```python
from build123d import *

# Parameters (mm, degrees)
RESSALTO_EXTRUS_O1_DEPTH = 1.4
ESBO_O2_R                = 3.45
RESSALTO_EXTRUS_O2_DEPTH = 2.4
FURO4_D                  = 1.2
PADR_O_LINEAR1_COUNT     = 6
PADR_O_LINEAR1_PITCH     = 2
FURO1_D                  = 4.95
FURO1_DEPTH              = 2
FURO2_D                  = 4.6
FURO2_DEPTH              = 1
FURO3_D                  = 2.1


with BuildPart() as part:
    # Esboço1 → Ressalto-extrusão1 (new body)
    with BuildSketch(Plane(origin=(0, 0, 0), x_dir=(1, 0, 0), z_dir=(0, 1, 0))):
        with BuildLine():
            Line((-14.159121967, 1.99702088), (-2.209072203, 2.65))
            ThreePointArc((-2.209072203, 2.65), (3.45, 0), (-2.209072203, -2.65))
            Line((-2.209072203, -2.65), (-14.159121967, -1.99702088))
            ThreePointArc((-14.159121967, -1.99702088), (-16.05, 0), (-14.159121967, 1.99702088))
        make_face()
    extrude(amount=-RESSALTO_EXTRUS_O1_DEPTH)

    # Esboço2 → Ressalto-extrusão2 (add)
    with BuildSketch(Plane.XZ.offset(1.4)):
        with Locations(Location((0, 0, 0), (0, 0, 90))):
            Circle(ESBO_O2_R)
    extrude(amount=RESSALTO_EXTRUS_O2_DEPTH)

    # Furo4 (through all)
    with Locations(Plane(origin=(0, 0, 0), x_dir=(1, 0, 0), z_dir=(0, 1, 0))):
        with Locations((-14.45, 0)):
            furo4 = Hole(FURO4_D / 2)

    # Padrão linear1: Furo4 ×6
    with Locations(*[(i * PADR_O_LINEAR1_PITCH, 0, 0) for i in range(1, PADR_O_LINEAR1_COUNT)]):
        add(furo4, mode=Mode.SUBTRACT)

    # Furo1
    with Locations(Plane(origin=(0, -3.8, 0), x_dir=(-1, 0, 0), z_dir=(0, -1, 0))):
        with Locations((0, 0)):
            Hole(FURO1_D / 2, depth=FURO1_DEPTH)

    # Furo2
    with Locations(Plane(origin=(0, 0, 0), x_dir=(1, 0, 0), z_dir=(0, 1, 0))):
        with Locations((0, 0)):
            Hole(FURO2_D / 2, depth=FURO2_DEPTH)

    # Furo3 (through all)
    with Locations(Plane(origin=(0, 0, 0), x_dir=(1, 0, 0), z_dir=(0, 1, 0))):
        with Locations((0, 0)):
            Hole(FURO3_D / 2)


solid = part.part
```
Here's how the part is built. I have some questions about the finished solid (model axes, mm). A direction names the side the tool comes from. Coordinates: 2 decimals unless noted, no trailing zeros. Order: outer loops, then holes, each group sorted by start corner. A loop starts at its lowest first (then second) coordinate and runs counter-clockwise, first axis right, second up. Notation, with made-up numbers: (86.25, 30.5) -> (137.25, 30.5) arc R4 cw to (137.25, 35.5) -> close; hole circle Ø8 at (43, 32). An arc over 180 degrees is marked (long way). Return JSON: item names as keys, results as strings.
1) If we section it at B-B on x = -6.45: List the corners of the cut face in (y, z) for me, plus the area to 3 significant figures.
Conclusion:
{"outline": "(-1.4, -2.42) -> (0, -2.42) -> (0, -0.6) -> (-1.4, -0.6) -> close; (-1.4, 0.6) -> (0, 0.6) -> (0, 2.42) -> (-1.4, 2.42) -> close", "area": "5.09 mm²"}
2) If we section it at D-D on z = 1.25: List the corners of the cut face in (x, y) for me, plus the area to 3 significant figures.
Conclusion:
{"outline": "(-15.61, -1.4) -> (-3.22, -1.4) -> (-3.22, -3.8) -> (-2.14, -3.8) -> (-2.14, -1.8) -> (2.14, -1.8) -> (2.14, -3.8) -> (3.22, -3.8) -> (3.22, 0) -> (1.93, 0) -> (1.93, -1) -> (-1.93, -1) -> (-1.93, 0) -> (-15.61, 0) -> close", "area": "29.4 mm²"}
3) If I drill on probe 1 along Z at (x, y) = (0, -0.2); probe 2 along Y at (x, z) = (1.5, 1); probe 3 along X at (y, z) = (-3.6, -1.25), over which ranges is the centre line in solid material (lowest first)?
Conclusion:
{"probe 1": "z = -3.45 to -2.3, 2.3 to 3.45", "probe 2": "y = -1.8 to -1", "probe 3": "x = -3.22 to -2.14, 2.14 to 3.22"}
4) Thinking about a two-plate mould opening in Z: for faces 4 (the cylindrical face through (2.36, -2.79, -0.74)), 5 (the cylindrical face through (-16.05, -0.69, 0.04)), 6 (the flat face through (-9, -1.4, 1)), 7 (the cylindrical face through (-15.004, -0.71, 0.23)), which applies, +Z half, -Z half, draft (parallel to the pull), parting line (faces both ways), or undercut?
Conclusion:
{"face 4": "undercut", "face 5": "parting line", "face 6": "draft", "face 7": "undercut"}
5) On a 3-axis mill with a long thin cutter (end or side, diameter ignored), from which of +Z, -Z, +X, -X, +Y, -Y can I reach the whole of each face in a straight line? I mean faces 1 (the cylindrical face through (-9.004, -0.71, 0.23)), 2 (the flat face through (1, -1.8, 1)), 3 (the cylindrical face through (1.825, -0.507, 1.4)). Say none if no direction works.
Conclusion:
{"face 1": "+Y, -Y", "face 2": "-Y", "face 3": "+Y"}
6) If we section it at A-A on y = -0.3: List the corners of the cut face in (x, z) for me, plus the area to 3 significant figures.
Conclusion:
{"outline": "(-14.16, -2) -> (-2.21, -2.65) arc R3.45 ccw (long way) to (-2.21, 2.65) -> (-14.16, 2) arc R2 ccw to start; hole circle Ø1.2 at (-14.45, 0); hole circle Ø1.2 at (-12.45, 0); hole circle Ø1.2 at (-10.45, 0); hole circle Ø1.2 at (-8.45, 0); hole circle Ø1.2 at (-6.45, 0); hole circle Ø1.2 at (-4.45, 0); hole circle Ø4.6 at (0, 0)", "area": "70.8 mm²"}
7) I'm going to push flat-ended pins straight in: P1, Ø1.4, axis at x = -10.45, z = 0, coming from the -Y side; P2, Ø1, axis at x = -4.45, z = 0, coming from the +Y side; P3, Ø3.5, axis at x = 0, z = 0, coming from the -Y side; P4, Ø1, axis at x = -10, y = -1.5, coming from the +Z side. Where does each tip first touch, or does it pass through?
Conclusion:
{"P1": "stops at y = -1.4", "P2": "passes through", "P3": "stops at y = -1.8", "P4": "stops at z = 2.25"}
8) If we section it at C-C on y = -2.75: List the corners of the cut face in (x, z) for me (3 decimals), plus the area to 3 significant figures.
Conclusion:
{"outline": "circle Ø6.9 at (0, 0); hole circle Ø4.95 at (0, 0)", "area": "18.1 mm²"}
